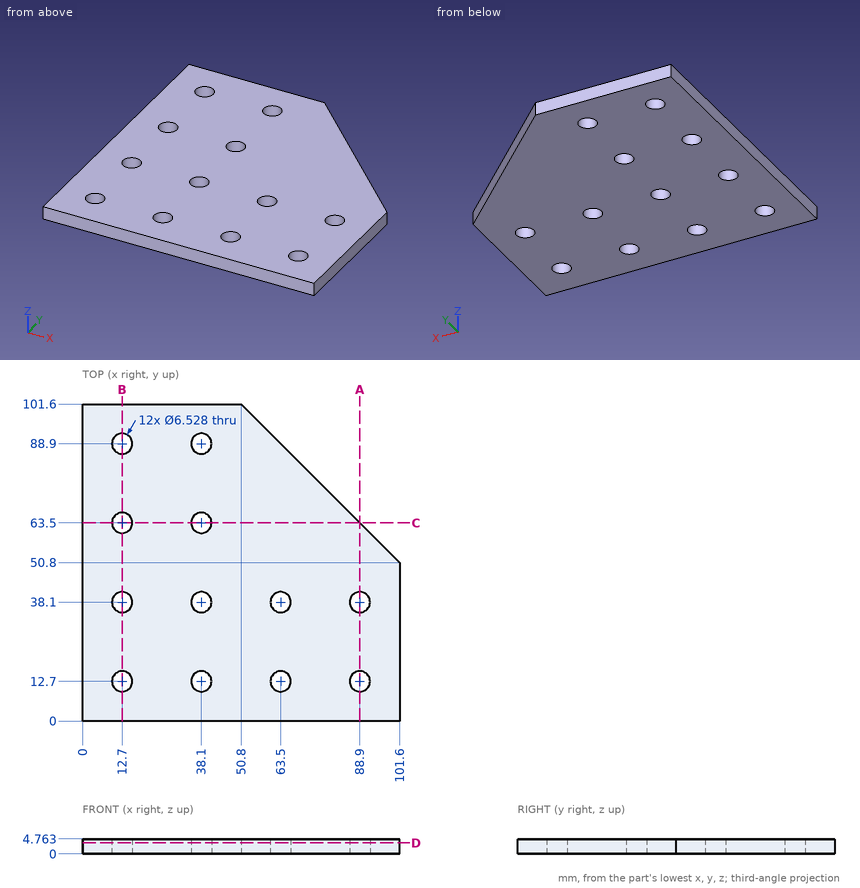
Part print with two shaded views. Sizes in mm from the minimum x, y, z corner. Round coordinates to 2 decimals unless told otherwise and drop trailing zeros. Order: outer loops, then holes, each group sorted by start corner. A loop starts at its lowest first (then second) coordinate and runs counter-clockwise, first axis right, second up. Notation, with made-up numbers: (-15.75, 38.25) -> (25.25, 38.25) arc R12 ccw to (25.25, 48.25) -> close; hole circle Ø11 at (-14.5, 38.5). An arc over 180 degrees is marked (long way). Use one line per item in the form item = value.
Item 1: Drill centre lines: line 1 (Y direction, x = 38.1, z = 1.3); line 2 (Y direction, x = 66, z = 2.15) (1 decimal); line 3 (Y direction, x = 63, z = 3.85) (1 decimal). Where is each one in solid material? Low to high.
Returned:
line_1 = 0 to 9.44, 15.96 to 34.84, 41.36 to 60.24, 66.76 to 85.64, 92.16 to 101.6
line_2 = 0 to 10.6, 14.8 to 36, 40.2 to 86.4
line_3 = 0 to 9.5, 15.9 to 34.9, 41.3 to 89.4
Item 2: Cut at B-B, the plane x = 12.7. Write the cut outline in (y, z).
Returned:
outline = (0, 0) -> (9.44, 0) -> (9.44, 4.76) -> (0, 4.76) -> close; (15.96, 0) -> (34.84, 0) -> (34.84, 4.76) -> (15.96, 4.76) -> close; (41.36, 0) -> (60.24, 0) -> (60.24, 4.76) -> (41.36, 4.76) -> close; (66.76, 0) -> (85.64, 0) -> (85.64, 4.76) -> (66.76, 4.76) -> close; (92.16, 0) -> (101.6, 0) -> (101.6, 4.76) -> (92.16, 4.76) -> close
Item 3: Cut at A-A, the plane x = 88.9. Write the cut outline in (y, z), and give its area (3 significant figures).
Returned:
outline = (0, 0) -> (9.44, 0) -> (9.44, 4.76) -> (0, 4.76) -> close; (15.96, 0) -> (34.84, 0) -> (34.84, 4.76) -> (15.96, 4.76) -> close; (41.36, 0) -> (63.5, 0) -> (63.5, 4.76) -> (41.36, 4.76) -> close
area = 240 mm^2
Item 4: Cut at C-C, the plane y = 63.5. Write the cut outline in (x, z), and give its area (3 significant figures).
Returned:
outline = (0, 0) -> (9.44, 0) -> (9.44, 4.76) -> (0, 4.76) -> close; (15.96, 0) -> (34.84, 0) -> (34.84, 4.76) -> (15.96, 4.76) -> close; (41.36, 0) -> (88.9, 0) -> (88.9, 4.76) -> (41.36, 4.76) -> close
area = 361 mm^2
Item 5: Cut at D-D, the plane z = 3.5. Give the number of separate pieces and of enclosed holes in the cut face, and give its area (3 significant figures).
Returned:
separate_pieces = 1
enclosed_holes = 12
area = 8,630 mm^2
Item 6: Flat gauge pins, fed straight in: pin 1 Ø4 at (x, y) = (12.7, 38.1) entering from -Z; pin 2 Ø7.5 at (x, y) = (38.1, 12.7) entering from -Z. Where does each tip first touch, or does it go through?
Returned:
pin_1 = through
pin_2 = 0
